Can you work these out from the drawing? Everything is in mm from the part's minimum corner. A direction names the side the tool comes from. Coordinates: 2 decimals unless noted, no trailing zeros. Loops run counter-clockwise (first coordinate to the right, second up) from the corner with the lowest first, then second, coordinate; pieces in that order, holes last. Notation, with made-up numbers: (-25, 45.5) - (23, 45.5) arc R26 cw to (23, 65.5) - close; hole circle Ø10 at (53, -22). An arc over 180 degrees is marked (long way). One line per question, with ' | ' between items. Start each with the question number.
1. I'm going to push flat-ended pins straight in: P1, Ø5, axis at x = 5.5, z = 11.5, coming from the +Y side; P2, Ø3, axis at x = 8.5, z = 11, coming from the -Y side; P3, Ø4, axis at x = 17, y = 14.5, coming from the +Z side. Where does each tip first touch, or does it pass through?
2. Please list where these lines run through material, in increasing order: L1, parallel to X at y = 15.75, z = 37.5; L2, parallel to Z at x = 9.75, y = 14.5; L3, parallel to Y at x = 19.5, z = 23. Write a range as [from, to].
3. I want a section at C-C, the plane y = 5.25. Write out the boundary of the cut face in (x, z).
4. I want a section at B-B, the plane z = 6. Write out the boundary of the cut face in (x, y), then the cut area to 3 significant figures.
5. I want a section at D-D, the plane x = 12.5. Write out the boundary of the cut face in (y, z).
6. We'd pull the mould along X, two halves only. Please class the marked faces 1, 2, 3 and 4: pulls with the +X half, pulls with the -X half, needs draft (parallel to the pull), parting line crosses it, or undercut.
7. Which directions (+Z, -Z, +X, -X, +Y, -Y) give clear straight access to the entire face, cutting with the end or side of a thin tool? Please do the marked faces 5 and 6.
8. I want a section at A-A, the plane x = 5.5. Write out the boundary of the cut face in (y, z).
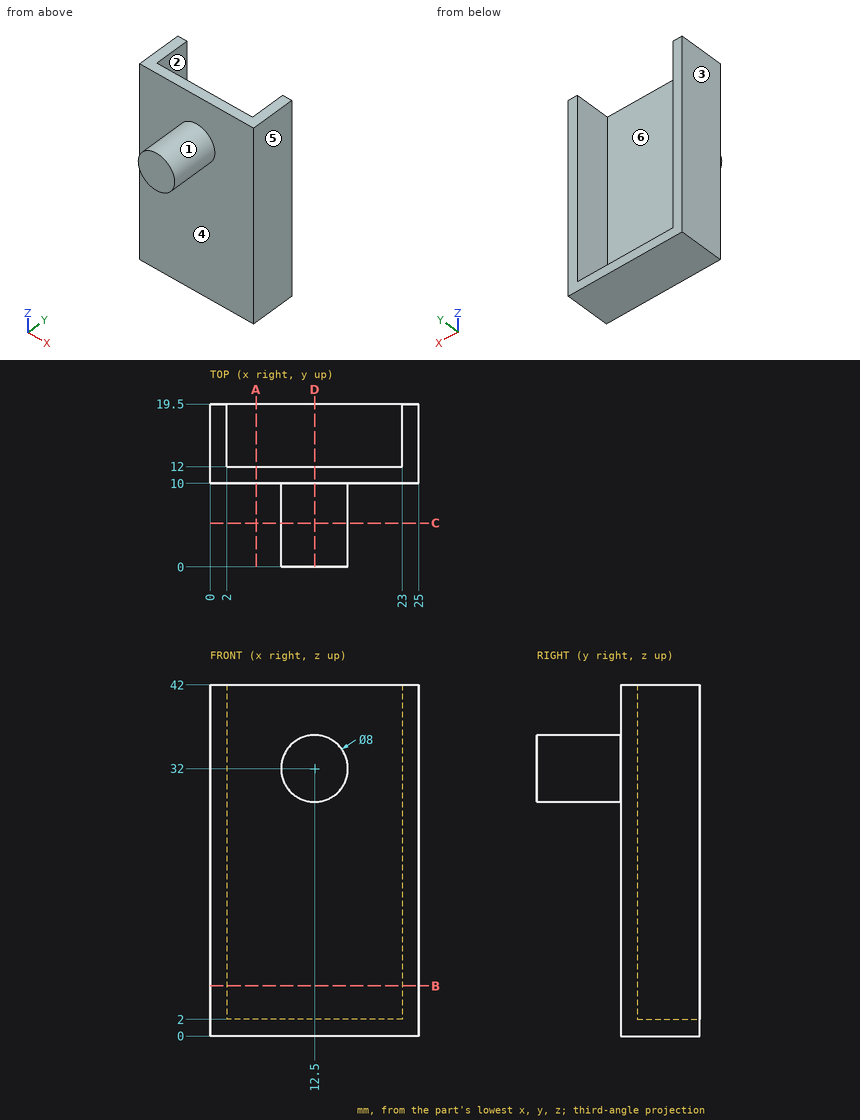
Results are:
1) P1: stops at y = 12 | P2: stops at y = 10 | P3: stops at z = 2
2) L1: x = [0, 2], [23, 25] | L2: z = [0, 2] | L3: y = [10, 12]
3) outline: circle Ø8 at (12.5, 32)
4) outline: (0, 10) - (25, 10) - (25, 19.5) - (23, 19.5) - (23, 12) - (2, 12) - (2, 19.5) - (0, 19.5) - close | area: 80.0 mm2
5) outline: (0, 28) - (10, 28) - (10, 0) - (19.5, 0) - (19.5, 2) - (12, 2) - (12, 42) - (10, 42) - (10, 36) - (0, 36) - close
6) face 1: parting line crosses it | face 2: undercut | face 3: pulls with the -X half | face 4: needs draft
7) face 5: +Z, -Z, +X, +Y, -Y | face 6: +Z, +Y
8) outline: (10, 0) - (19.5, 0) - (19.5, 2) - (12, 2) - (12, 42) - (10, 42) - close
